Input: part model. Units: mm. Frame: model coordinates. A direction names the side the tool comes from. Give positions to 0.01 mm unless a question says otherwise; leave off trailing zeros. Loops run counter-clockwise (first coordinate to the right, second up) from the corner with the lowest first, then second, coordinate; pieces in that order, holes last.
from build123d import *

# Parameters (mm, degrees)
SKETCH1_R           = 120
BOSS_EXTRUDE2_DEPTH = 10
SKETCH2_R           = 117.5
BOSS_EXTRUDE3_DEPTH = 7.5
SKETCH3_R           = 120
BOSS_EXTRUDE4_DEPTH = 10
SKETCH4_R           = 117.5
BOSS_EXTRUDE5_DEPTH = 7.5
SKETCH5_R           = 120
BOSS_EXTRUDE6_DEPTH = 10
SKETCH6_R           = 18.75
CUT_EXTRUDE1_DEPTH  = 50


with BuildPart() as part:
    # Sketch1 → Boss-Extrude2 (new body)
    with BuildSketch(Plane.XY):
        Circle(SKETCH1_R)
    extrude(amount=BOSS_EXTRUDE2_DEPTH)

    # Sketch2 → Boss-Extrude3 (add)
    with BuildSketch(Plane.XY.offset(10)):
        Circle(SKETCH2_R)
    extrude(amount=BOSS_EXTRUDE3_DEPTH)

    # Sketch3 → Boss-Extrude4 (add)
    with BuildSketch(Plane.XY.offset(17.5)):
        Circle(SKETCH3_R)
    extrude(amount=BOSS_EXTRUDE4_DEPTH)

    # Sketch4 → Boss-Extrude5 (add)
    with BuildSketch(Plane.XY.offset(27.5)):
        Circle(SKETCH4_R)
    extrude(amount=BOSS_EXTRUDE5_DEPTH)

    # Sketch5 → Boss-Extrude6 (add)
    with BuildSketch(Plane.XY.offset(35)):
        Circle(SKETCH5_R)
    extrude(amount=BOSS_EXTRUDE6_DEPTH)

    # Sketch6 → Cut-Extrude1 (cut)
    with BuildSketch(Plane.XY.offset(45)):
        Circle(SKETCH6_R)
    extrude(amount=-CUT_EXTRUDE1_DEPTH, mode=Mode.SUBTRACT)


solid = part.part
(1) Cut plane D-D (x = 77). Return the cut outline in (y, z).
Values follow:
outline: (-92.04, 0) - (92.04, 0) - (92.04, 10) - (88.75, 10) - (88.75, 17.5) - (92.04, 17.5) - (92.04, 27.5) - (88.75, 27.5) - (88.75, 35) - (92.04, 35) - (92.04, 45) - (-92.04, 45) - (-92.04, 35) - (-88.75, 35) - (-88.75, 27.5) - (-92.04, 27.5) - (-92.04, 17.5) - (-88.75, 17.5) - (-88.75, 10) - (-92.04, 10) - close
(2) Cut plane C-C (z = 14.5). Return the cut outline in (x, y), and give its area (3 significant figures).
Values follow:
outline: circle Ø235 at (0, 0); hole circle Ø37.5 at (0, 0)
area: 42,300 mm2
(3) Cut plane A-A (x = 0). Return the cut outline in (y, z), and give its area (3 significant figures).
Values follow:
outline: (-120, 0) - (-18.75, 0) - (-18.75, 45) - (-120, 45) - (-120, 35) - (-117.5, 35) - (-117.5, 27.5) - (-120, 27.5) - (-120, 17.5) - (-117.5, 17.5) - (-117.5, 10) - (-120, 10) - close; (18.75, 0) - (120, 0) - (120, 10) - (117.5, 10) - (117.5, 17.5) - (120, 17.5) - (120, 27.5) - (117.5, 27.5) - (117.5, 35) - (120, 35) - (120, 45) - (18.75, 45) - close
area: 9,040 mm2
(4) Pin query (flat end, axial travel): pin 1 Ø4 at (y, z) = (54, 10.5) entering from -X; pin 2 Ø6 at (y, z) = (-87.5, 14) entering from +X; pin 3 Ø1.5 at (y, z) = (62, 9.5) entering from +X; pin 4 Ø1 at (x, y) = (37, -28) entering from -Z. Return the tip coordinate at first contact, or that it passes through.
Values follow:
pin 1: stops at x = -108.12
pin 2: stops at x = 81.65
pin 3: stops at x = 103.19
pin 4: stops at z = 0
(5) Ray query, probe 1 along Y at (x, z) = (0, 16); probe 2 along X at (y, z) = (10, 16); probe 3 along X at (y, z) = (15.5, 37). Return the intervals inside material, ascending.
Values follow:
probe 1: y = -117.5 to -18.75, 18.75 to 117.5
probe 2: x = -117.07 to -15.86, 15.86 to 117.07
probe 3: x = -118.99 to -10.55, 10.55 to 118.99
(6) Mould query, pull axis Z, two halves, no side actions, for faces 3 (the flat face through (88, -79, 17.5)), 4 (the cylindrical face through (-119.884, 5.276, 22.43)), 5 (the flat face through (25, 2, 45)), 6 (the cylindrical face through (-15.3, 116.5, 31.2)). Classes: +Z half, -Z half, draft (parallel to the pull), parting line (faces both ways), or undercut.
Values follow:
face 3: undercut
face 4: draft
face 5: +Z half
face 6: undercut
(7) Reachability of faces 1 (the cylindrical face through (-119.884, 5.276, 39.93)), 2 (the cylindrical face through (-15.3, 116.5, 13.7)) from +Z, -Z, +X, -X, +Y, -Y: full face, straight path, thin tool, end or side. Return the list, or none.
Values follow:
face 1: +Z, -Z
face 2: none
